Can you work these out from the model? Positions are in its coordinate system, mm. Coordinates: 2 decimals unless noted, no trailing zeros. Loops run counter-clockwise (first coordinate to the right, second up) from the corner with the lowest first, then second, coordinate; pieces in that order, holes last.
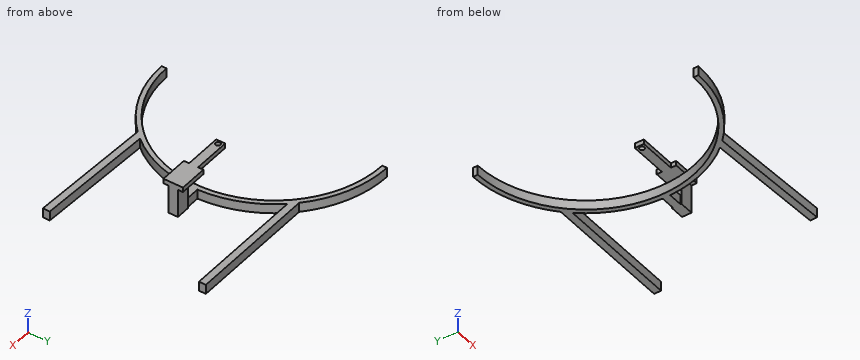
```python
from build123d import *

# Parameters (mm, degrees)
SKETCH1_R           = 2.5
BOSS_EXTRUDE1_DEPTH = 5
SKETCH2_W           = 15
SKETCH2_H           = 10
BOSS_EXTRUDE2_DEPTH = 30
SKETCH3_W           = 10
SKETCH3_H           = 8
BOSS_EXTRUDE3_DEPTH = 20
BOSS_EXTRUDE5_DEPTH = 10
BOSS_EXTRUDE6_DEPTH = 10


with BuildPart() as part:
    # Sketch1 → Boss-Extrude1 (new body)
    with BuildSketch(Plane.XY):
        Polygon((-15, 4.74891783), (-15, 10.327635328), (15, 10.327635328), (15, -10.327635328), (-15, -10.327635328), (-15, -4.74891783), (-55, -4.74891783), (-55, 4.74891783), align=None)
        with Locations((-51, 0)):
            Circle(SKETCH1_R, mode=Mode.SUBTRACT)
    extrude(amount=BOSS_EXTRUDE1_DEPTH)

    # Sketch2 → Boss-Extrude2 (add)
    with BuildSketch(Plane(origin=(0, 0, 0), x_dir=(-1, 0, 0), z_dir=(0, 0, -1))):
        with Locations((-7.5, 0)):
            Rectangle(SKETCH2_W, SKETCH2_H)
    extrude(amount=BOSS_EXTRUDE2_DEPTH)

    # Sketch3 → Boss-Extrude3 (add)
    with BuildSketch(Plane.ZY):
        with Locations((-25, 0)):
            Rectangle(SKETCH3_W, SKETCH3_H)
    extrude(amount=BOSS_EXTRUDE3_DEPTH)

    # Sketch5 → Boss-Extrude5 (add)
    with BuildSketch(Plane(origin=(0, 0, -30), x_dir=(-1, 0, 0), z_dir=(0, 0, -1))):
        with BuildLine():
            Line((134, -114), (134, -119))
            ThreePointArc((134, -119), (15, 0), (134, 119))
            Line((134, 119), (134, 114))
            ThreePointArc((134, 114), (20, 0), (134, -114))
        make_face()
    extrude(amount=-BOSS_EXTRUDE5_DEPTH)

    # Sketch6 → Boss-Extrude6 (add)
    with BuildSketch(Plane(origin=(0, 0, -30), x_dir=(-1, 0, 0), z_dir=(0, 0, -1))):
        with BuildLine():
            Line((51.28059478, 85.54823201), (-86.273042092, 85.54823201))
            Line((-86.273042092, 85.54823201), (-86.273042092, 78.202780321))
            Line((-86.273042092, 78.202780321), (44.304263479, 78.202780321))
            ThreePointArc((44.304263479, 78.202780321), (47.714229501, 81.94977614), (51.28059478, 85.54823201))
        make_face()
        with BuildLine():
            Line((-83.044588659, -81.622968191), (47.426200609, -76.349840264))
            ThreePointArc((47.426200609, -76.349840264), (50.984700645, -79.956074232), (54.69347384, -83.407573519))
            Line((54.69347384, -83.407573519), (-82.7479559, -88.962427947))
            Line((-82.7479559, -88.962427947), (-83.044588659, -81.622968191))
        make_face()
    extrude(amount=-BOSS_EXTRUDE6_DEPTH)


solid = part.part
```
(1) I want a section at C-C on x = 18.5. Write out the boundary of the cut face in (y, z).
Check values:
outline: (-86.37, -30) - (-79.01, -30) - (-79.01, -20) - (-86.37, -20) - close; (78.2, -30) - (85.55, -30) - (85.55, -20) - (78.2, -20) - close
(2) If I drill on probe 1 along Y at (x, z) = (-51, 1.8); probe 2 along X at (y, z) = (-1.5, -7); probe 3 along Y at (x, z) = (0.5, -10), over which ranges is the centre line in solid material (lowest first)?
Check values:
probe 1: y = -4.75 to -2.5, 2.5 to 4.75
probe 2: x = 0 to 15
probe 3: y = -5 to 5
(3) I want a section at B-B on z = -27. Write out the boundary of the cut face in (x, y), then the cut area to 3 significant figures.
Check values:
outline: (-134, -119) arc R119 ccw to (-49.34, -83.62) - (82.75, -88.96) - (83.04, -81.62) - (-42.88, -76.53) arc R119 ccw to (-15.07, -4) - (0, -4) - (0, -5) - (15, -5) - (15, 5) - (0, 5) - (0, 4) - (-15.07, 4) arc R119 ccw to (-44.3, 78.2) - (86.27, 78.2) - (86.27, 85.55) - (-51.28, 85.55) arc R119 ccw to (-134, 119) - (-134, 114) arc R114 cw to (-134, -114) - close
area: 4,030 mm2
(4) I want a section at A-A on x = -72. Write out the boundary of the cut face in (y, z), then the cut area to 3 significant figures.
Check values:
outline: (-101.57, -30) - (-95.67, -30) - (-95.67, -20) - (-101.57, -20) - close; (95.67, -30) - (101.57, -30) - (101.57, -20) - (95.67, -20) - close
area: 118 mm2
(5) I want a section at D-D on y = -102.5. Write out the boundary of the cut face in (x, z).
Check values:
outline: (-84.1, -30) - (-73.55, -30) - (-73.55, -20) - (-84.1, -20) - close
(6) I'm going to push flat-ended pins straight in: pin 1 (12 mm diameter, centred on x = 6.5, z = -10, fed in from +Y); pin 2 (4 mm diameter, centred on y = 7, z = 1.5, fed in from -X); pin 3 (2.5 mm diameter, centred on x = 6.5, z = 1.5, fed in from -Y); pin 4 (3 mm diameter, centred on x = -51, y = 0, fed in from -Z). Where does each tip first touch, or does it pass through?
Check values:
pin 1: stops at y = 5
pin 2: stops at x = -15
pin 3: stops at y = -10.33
pin 4: passes through
